Answer from the drawing. Dimensions are ordinates in mm from the lowest x, y and z of the part. A direction names the side the tool comes from. Give positions to 0.01 mm unless a question says otherwise; leave off trailing zeros. Order: outer loops, then holes, each group sorted by start corner. A loop starts at its lowest first (then second) coordinate and runs counter-clockwise, first axis right, second up.
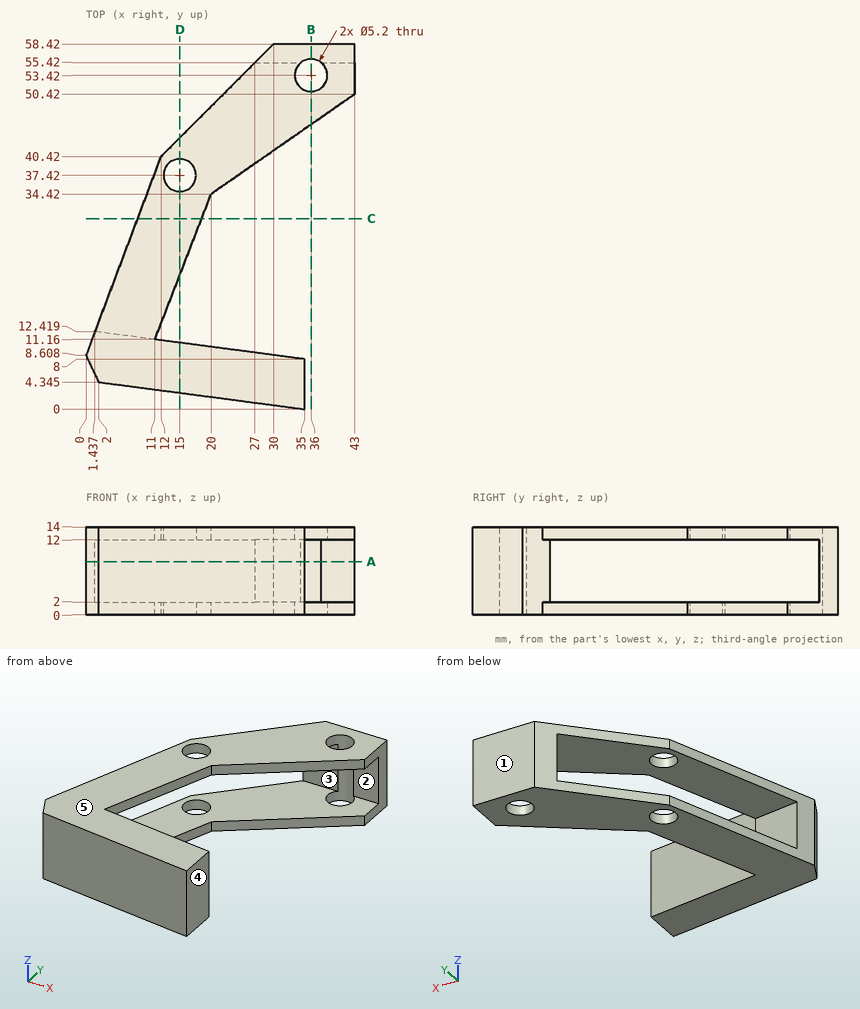
1) The part is cut by section B-B on x = 36. Determine the outline of the cut face in (y, z).
Final values:
outline: (45.55, 0) - (50.82, 0) - (50.82, 2) - (45.55, 2) - close; (45.55, 12) - (50.82, 12) - (50.82, 14) - (45.55, 14) - close; (56.02, 0) - (58.42, 0) - (58.42, 14) - (56.02, 14) - close
2) A tool of negligible diameter and unlimited length cuts with its end or side. For the marked faces 1 and 2, from which of +Z, -Z, +X, -X, +Y, -Y can it reach the whole face along a straight path? Write none if from no direction.
Final values:
face 1: +Z, -Z, +X, -X, +Y
face 2: +X, -X, -Y
3) Given pin 1 (1.6 mm diameter, centred on x = 39, z = 8.5, fed in from -Y); pin 2 (8 mm diameter, centred on x = 30, z = 7, fed in from -Y); pin 3 (4 mm diameter, centred on y = 3, z = 4.5, fed in from +X), each flat-ended and moving along its own axis, determine where each tip first touches the part or whether it passes through.
Final values:
pin 1: stops at y = 55.42
pin 2: stops at y = 0.13
pin 3: stops at x = 35
4) The part is cut by section D-D on x = 15. Determine the outline of the cut face in (y, z), and give its area (3 significant figures).
Final values:
outline: (2.63, 0) - (10.63, 0) - (10.63, 14) - (2.63, 14) - close; (21.5, 0) - (34.82, 0) - (34.82, 2) - (21.5, 2) - close; (21.5, 12) - (34.82, 12) - (34.82, 14) - (21.5, 14) - close; (40.02, 0) - (43.42, 0) - (43.42, 2) - (40.02, 2) - close; (40.02, 12) - (43.42, 12) - (43.42, 14) - (40.02, 14) - close
area: 179 mm2
5) For a pull along Z with two mould halves and no side action, classify the marked faces 3, 4 and 5 as released by +Z, released by -Z, zero draft, split by the parting line, or undercut.
Final values:
face 3: undercut
face 4: zero draft
face 5: released by +Z
6) The part is cut by section C-C on y = 30.5. Determine the outline of the cut face in (x, z).
Final values:
outline: (8.26, 0) - (18.48, 0) - (18.48, 2) - (8.26, 2) - close; (8.26, 12) - (18.48, 12) - (18.48, 14) - (8.26, 14) - close
7) Consider L1, parallel to Z at x = 18, y = 45; L2, parallel to Y at x = 41, z = 6.5; L3, parallel to Y at x = 29, z = 1.5. Determine where each line is inside the solid, lowest interval first.
Final values:
L1: z = 0 to 2, 12 to 14
L2: y = 55.42 to 58.42
L3: y = 0.79 to 8.79, 40.68 to 57.42
8) The part is cut by section A-A on z = 8.5. Determine the outline of the cut face in (x, y) (1 decimal), and give its area (3 significant figures).
Final values:
outline: (0, 8.6) - (2, 4.3) - (35, 0) - (35, 8) - (1.4, 12.4) - close; (27, 55.4) - (34.3, 55.4) arc R2.6 cw to (37.7, 55.4) - (43, 55.4) - (43, 58.4) - (30, 58.4) - close
area: 315 mm2
